Autodesk Inventor part; units mm, degrees
ref_plane "YZ Plane" through (0, 0, 0) normal (1, 0, 0) x (0, 1, 0)
ref_plane "XZ Plane" through (0, 0, 0) normal (0, 1, 0) x (-1, 0, 0)
ref_plane "XY Plane" through (0, 0, 0) normal (0, 0, 1) x (1, 0, 0)
sketch "Skizze1" plane through (0, 0, 0) normal (0, 0, 1) x (1, 0, 0)
  line L0 (-14, 0) -> (14, 0)
  line L1 (0, -15.4) -> (0, 15.4)
  line L2 (-10, 11) -> (10, 11)
  line L3 (10, 11) -> (10, -11)
  line L4 (10, -11) -> (-10, -11)
  line L5 (-10, -11) -> (-10, 11)
  point P0 (0, 0)
  dimension "d0" = 22
  dimension "d1" = 20
extrude "Extrusion1" add sketch "Skizze1" along normal blind 37
sketch "Skizze2" plane through (0, 0, 0) normal (0, 0, -1) x (-1, 0, 0)
  point P0 (0, 0)
hole "Bohrung1" at (0, 0, 0) direction (0, 0, 1) diameter 12.5 depth 32 tip angle 118
sketch "Skizze3" plane through (0, 0, 0) normal (0, 0, -1) x (-1, 0, 0)
  line L0 (14, 0) -> (-14, 0)
  line L1 (0, -15.4) -> (0, 15.4)
  line L2 (-5.5, 6.5) -> (5.5, 6.5)
  line L3 (5.5, 6.5) -> (5.5, -6.5)
  line L4 (5.5, -6.5) -> (-5.5, -6.5)
  line L5 (-5.5, -6.5) -> (-5.5, 6.5)
  dimension "d11" = 13
  dimension "d12" = 11
extrude "Extrusion2" cut sketch "Skizze3" against normal blind 10
fillet "Rundung1" radius 1.5 4 edges at (-5.5, -6.5, 5) (-5.5, 6.5, 5) (5.5, 6.5, 5) (5.5, -6.5, 5)
sketch "Skizze4" plane through (0, 0, 37) normal (0, 0, 1) x (1, 0, 0)
  line L0 (-10, 11) -> (-10, -11)
  line L1 (-10, -11) -> (10, -11)
  line L2 (-4, -6.5) -> (4, -6.5)
  arc A0 (4, -6.5) -> (5.5, -5) centre (4, -5) ccw
  line L3 (5.5, -5) -> (5.5, -2.9686)
  arc A1 (-5.5, -5) -> (-4, -6.5) centre (-4, -5) ccw
  line L4 (-5.5, -2.9686) -> (-5.5, -5)
  line L5 (-10, -7) -> (-5, -7)
  line L6 (-5, -7) -> (-5, -11)
  line L7 (-5, -11) -> (-10, -11)
  line L8 (-10, -11) -> (-10, -7)
  line L9 (10, -11) -> (5, -11)
  line L10 (5, -11) -> (5, -7)
  line L11 (5, -7) -> (10, -7)
  line L12 (10, -7) -> (10, -11)
  point P0 (0, 0)
  dimension "d16" = 5
  dimension "d17" = 4
  dimension "d18" = 5
extrude "Extrusion3" cut sketch "Skizze4" against normal through all
fillet "Rundung2" radius 3 2 edges at (-5, -7, 18.5) (5, -7, 18.5)
sketch "Skizze5" plane through (-10, 11, 0) normal (0, 1, 0) x (1, 0, 0)
  line L0 (0, 0) -> (20, 0)
  line L1 (0, 0) -> (20, 0)
  line L2 (20, 0) -> (20, -10)
  line L3 (20, -10) -> (0, -10)
  line L4 (0, -10) -> (0, 0)
  line L5 (-4, 0) -> (24, 0)
  line L6 (10, 7.4) -> (10, -44.4)
  point P0 (10, 0)
  dimension "d22" = 20
  dimension "d23" = 10
extrude "Extrusion4" add sketch "Skizze5" along normal blind 10
sketch "Skizze7" plane through (0, 0, 0) normal (0, 0, -1) x (-1, 0, 0)
  circle A0 centre (-6, 9) radius 1.2
  circle A1 centre (6, 9) radius 1.2
  circle A2 centre (0, -9) radius 1.2
hole "Bohrung3" at (6, 9, 0) at (-6, 9, 0) at (0, -9, 0) direction (0, 0, 1) diameter 1.567 depth 6 tip angle 118
sketch "Skizze8" plane through (-10, 11, 37) normal (0, 1, 0) x (1, 0, 0)
  line L0 (20, 27) -> (0, 27)
  line L1 (0, 27) -> (0, 0)
  line L2 (20, 0) -> (0, 0)
  line L3 (20, 27) -> (20, 0)
  point P0 (10, 37)
extrude "Extrusion5" add sketch "Skizze8" along normal blind 6
sketch "Skizze9" plane through (-10, 21, 10) normal (0, 0, 1) x (1, 0, 0)
  line L0 (20, -4) -> (20, 0)
  line L1 (0, 0) -> (20, 0)
  circle A0 centre (4, -12) radius 1.2
  circle A1 centre (16, -12) radius 1.2
  circle A2 centre (10, -30) radius 1.2
  circle A3 centre (18, -1) radius 2.25
  circle A4 centre (18, -31) radius 2.25
  circle A5 centre (2, -31) radius 2.25
  circle A6 centre (2, -1) radius 2.25
  circle A7 centre (13, -17) radius 1.75
  circle A8 centre (7, -25) radius 1.75
  circle A9 centre (10, -25.5) radius 0.9
  circle A10 centre (10, -16.5) radius 0.9
  circle A11 centre (10, -21) radius 3
  line L2 (23, 2) -> (-3, 2)
  line L3 (-3, 2) -> (-3, -34)
  line L4 (-3, -34) -> (23, -34)
  line L5 (23, 2) -> (23, -34)
  line L6 (15, 0) -> (20, 0)
  line L7 (20, 0) -> (20, -4)
  line L8 (20, -4) -> (15, -4)
  line L9 (15, -4) -> (15, 0)
  line L10 (0, 0) -> (5, 0)
  line L11 (5, 0) -> (5, -4)
  line L12 (5, -4) -> (0, -4)
  line L13 (0, -4) -> (0, 0)
  line L14 (10, 0) -> (10, -17.7524)
  circle A12 centre (10, -12) radius 3
  point P0 (10, -21)
  dimension "d44" = 3
  dimension "d45" = 3
extrude "Extrusion6" cut sketch "Skizze9" against normal through all contours L8 L9 L1 A3 L0 | L11 L12 L13 A6 L1 | A3 L1 L0 | A6 L13 L1 picked at (17.2844, -1.2206) picked at (2.725, -1.1961)
fillet "Rundung3" radius 3 2 edges at (5, 17, 5) (-5, 17, 5)
sketch "Skizze10" plane through (0, 0, 0) normal (0, 0, -1) x (-1, 0, 0)
  line L0 (-5.5, -5) -> (-5.5, -2.9686)
  arc A0 (2, 11.2361) -> (-2, 11.2361) centre (0, 9) ccw
  arc A1 (-2, 11.2361) -> (2, 11.2361) centre (0, 9) ccw
  arc A2 (3, 9) -> (-3, 9) centre (0, 9) ccw
  line L1 (-3, 9) -> (-3, 4)
  line L2 (-3, 4) -> (3, 4)
  line L3 (3, 9) -> (3, 4)
  arc A3 (5.5, 2.9686) -> (-5.5, 2.9686) centre (0, 0) ccw
  dimension "d49" = 3
  dimension "d50" = 5
extrude "Extrusion7" cut sketch "Skizze10" against normal blind 32
sketch "Skizze11" plane through (-5, 21, 10) normal (0, 0, 1) x (1, 0, 0)
  line L0 (0, 0) -> (0, -1)
  arc A0 (-3, -4) -> (0, -1) centre (-3, -1) ccw
  line L1 (-3, -4) -> (13, -4)
  arc A1 (10, -1) -> (13, -4) centre (13, -1) ccw
  line L2 (10, -1) -> (10, 0)
  line L3 (0, 0) -> (10, 0)
  point P0 (5, -21)
extrude "Extrusion8" add sketch "Skizze11" along normal up to surface (27 mm away)
properties part number "13_1087_013" material "PPS-Kunststoff"
The listing builds one solid part. Answer for the finished solid, in the listing's coordinates (mm). A direction names the side the tool comes from. Round coordinates to 2 decimals unless told otherwise and drop trailing zeros. Loops run counter-clockwise (first coordinate to the right, second up) from the corner with the lowest first, then second, coordinate; pieces in that order, holes last. Notation, with made-up numbers: (34, 57) -> (59, 57) arc R14 ccw to (59, 65) -> close; hole circle Ø5 at (10.25, 81). An arc over 180 degrees is marked (long way). Use one line per item in the form item = value.
1. The part is cut by section C-C on z = 4. Give the number of separate pieces and of enclosed holes in the cut face, and give its area (3 significant figures).
Answer key:
separate_pieces = 1
enclosed_holes = 4
area = 386 mm²
2. A tool of negligible diameter and unlimited length cuts with its end or side. For faces 4 (the cylindrical face through (-5.07, -6.05, 5.07)), 5 (the flat face through (5, -10.5, 18.8)), 6 (the flat face through (9, 17, 18)), from which of +Z, -Z, +X, -X, +Y, -Y can it reach the whole face along a straight path? Write none if from no direction.
Answer key:
face_4 = -Z
face_5 = +Z, -Z, +X, -Y
face_6 = +Z, -Z, +X, +Y
3. The part is cut by section B-B on y = 7.5. Determine the outline of the cut face in (x, z), and give its area (3 significant figures).
Answer key:
outline = (-10, 0) -> (-3, 0) -> (-3, 32) -> (3, 32) -> (3, 0) -> (10, 0) -> (10, 37) -> (-10, 37) -> close
area = 548 mm²
4. For a pull along Y with two mould halves and no side action, classify faces 1 (the flat face through (0, 5, 37)), 2 (the conical face through (-5.87, 8.98, 6.39)), 3 (the cylindrical face through (5.9, 17.86, 18.24)) as released by +Y, released by -Y, zero draft, split by the parting line, or undercut.
Answer key:
face_1 = zero draft
face_2 = undercut
face_3 = released by +Y
5. Flat-ended cylindrical pins translate along their axes: pin 1 Ø0.6 at (x, z) = (9, 16.5) entering from +Y; pin 2 Ø1 at (x, z) = (9, 20) entering from -Y; pin 3 Ø1.8 at (x, y) = (-0.5, -4.5) entering from -Z. Find the tip coordinate at first contact, or state that the pin passes through.
Answer key:
pin_1 = 17
pin_2 = -7
pin_3 = 32.49
6. The part is cut by section D-D on y = -7.5. Determine the outline of the cut face in (x, z).
Answer key:
outline = (-6.34, 0) -> (6.34, 0) -> (6.34, 37) -> (-6.34, 37) -> close
7. Find the intervals of material crossed by probe 1 along Y at (x, z) = (0, 3.7); probe 2 along X at (y, z) = (9, 2); probe 3 along Y at (x, z) = (0, 12), in increasing order. Write a range as [from, to].
Answer key:
probe_1 = [-11, -9.78], [-8.22, -6.5], [12, 21]
probe_2 = [-10, -6.78], [-5.22, -3], [3, 5.22], [6.78, 10]
probe_3 = [-11, -6.25], [12, 21]
